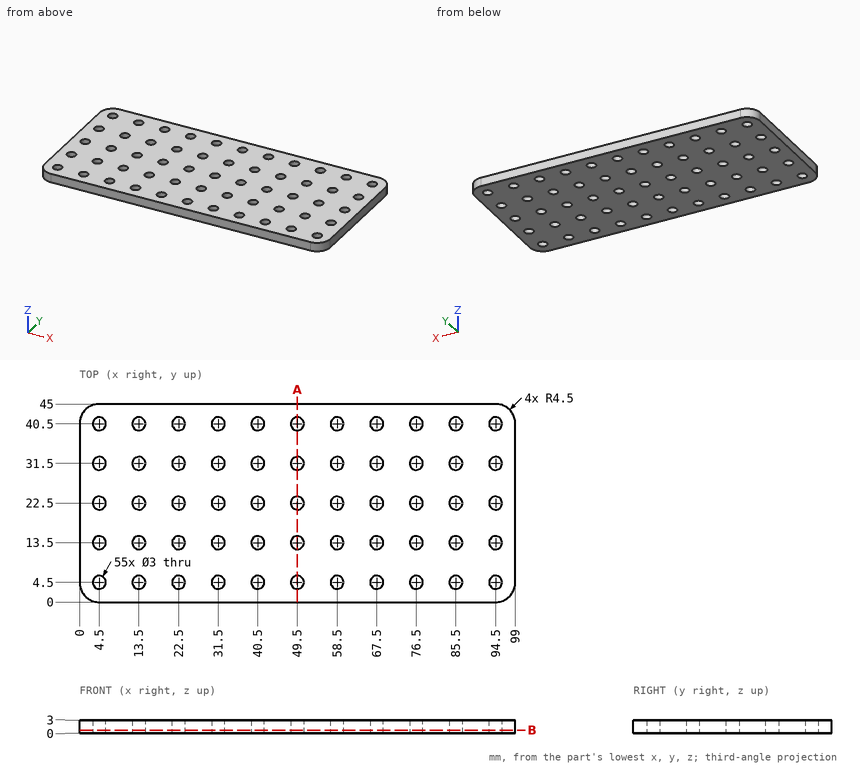
Geometry: see drawing. Coordinates: mm, zero at the bounding-box minimum. Coordinates: 2 decimals unless noted, no trailing zeros. Loops run counter-clockwise (first coordinate to the right, second up) from the corner with the lowest first, then second, coordinate; pieces in that order, holes last. Notation, with made-up numbers: (58.25, 18) - (64.25, 18) arc R22 cw to (64.25, 24) - close; hole circle Ø6 at (-15.75, -9.5). An arc over 180 degrees is marked (long way). Answer as CSV lines item,"result".
1. Section A-A (x = 49.5). Return loops of the section in (y, z), then the cut area to 3 significant figures.
Established:
outline,"(0, 0) - (3, 0) - (3, 3) - (0, 3) - close; (6, 0) - (12, 0) - (12, 3) - (6, 3) - close; (15, 0) - (21, 0) - (21, 3) - (15, 3) - close; (24, 0) - (30, 0) - (30, 3) - (24, 3) - close; (33, 0) - (39, 0) - (39, 3) - (33, 3) - close; (42, 0) - (45, 0) - (45, 3) - (42, 3) - close"
area,"90.0 mm2"
2. Section B-B (z = 0.75). Count the separate pieces of the cut face and the enclosed holes in it, then the cut area to 3 significant figures.
Established:
separate pieces,"1"
enclosed holes,"55"
area,"4,050 mm2"
3. Contact query for flat-ended pins moving along their axis: pin 1 (5 mm diameter, centred on x = 85.5, y = 13.5, fed in from +Z); pin 2 (1.8 mm diameter, centred on x = 49.5, y = 40.5, fed in from +Z). Output: stop coordinate, or through.
Established:
pin 1,"stops at z = 3"
pin 2,"passes through"
4. Ray query, line 1 (Y direction, x = 13.5, z = 1.95); line 2 (Y direction, x = 48.5, z = 1.3). Return the intervals inside material, ascending.
Established:
line 1,"y = 0 to 3, 6 to 12, 15 to 21, 24 to 30, 33 to 39, 42 to 45"
line 2,"y = 0 to 3.38, 5.62 to 12.38, 14.62 to 21.38, 23.62 to 30.38, 32.62 to 39.38, 41.62 to 45"
